Build history of the part. All positions in model axes, mm. A direction names the side the tool comes from. Round coordinates to 2 decimals unless told otherwise and drop trailing zeros. Write each loop counter-clockwise with the first axis right and the second up, starting at its lowest first coordinate (ties: lowest second). Pieces come first, ordered by that corner, then holes. Notation, with made-up numbers: (11.5, -7) - (31.5, -7) arc R35 cw to (31.5, 30) - close; hole circle Ø6 at (-32.75, 41). An arc over 180 degrees is marked (long way). Answer as a JSON object with one key per item and string values. Group by question number.
Item 1: Slice it at B-B, the plane z = -8. List the corners of the cut face in (x, y), then the cut area to 3 significant figures.
Item 2: Flat gauge pins, fed straight in: pin 1 (3 mm diameter, centred on x = 1, z = -7, fed in from +Y); pin 2 (2.5 mm diameter, centred on x = -0.5, z = -57.5, fed in from -Y); pin 3 (2 mm diameter, centred on x = 0, z = -58, fed in from -Y). Where does each tip first touch, or does it go through?
Item 3: Two-plate mould, pull along X, no slides. Class faces 4 (the cylindrical face through (0.07, 4.96, -73.7)), 5 (the flat face through (-5, 10, -41)): +X half, -X half, draft (parallel to the pull), parting line (faces both ways), or undercut.
Item 4: Slice it at A-A, the plane y = 1.25. List the corners of the cut face in (x, z), then the cut area to 3 significant figures.
Item 5: Probe line 1 (Z direction, x = 0, y = 9.25); line 2 (Y direction, x = -1.25, z = -30); line 3 (Z direction, x = 1.5, y = 9.25). List the from-to ranges inside material, lowest first. Write a range as from..to.
Item 6: Slice it at C-C, the plane x = 0. Give the number of separate pieces and of enclosed holes in the cut face, then the cut area to 3 significant figures.
Item 7: Slice it at D-D, the plane z = -30. List the corners of the cut face in (x, y).
Item 8: Which spindle directions (+Z, -Z, +X, -X, +Y, -Y) get a long thin tool onto all of the face, cutting with end or side? Do faces 1 (the cylindrical face through (0.07, 4.96, -59.7)), 2 (the cylindrical face through (0.103, 1.232, -74.348)), 3 (the flat face through (-3.44, 7.54, -37.96)). Say none if no direction does.
from build123d import *

# Parameters (mm, degrees)
SKETCH1_W           = 16
SKETCH1_H           = 80
BOSS_EXTRUDE1_DEPTH = 10
SKETCH2_R           = 2.35
CUT_EXTRUDE1_DEPTH  = 2.5
SKETCH2_3_R         = 1.7
CUT_EXTRUDE2_DEPTH  = 82.018516402
CUT_EXTRUDE3_START  = 7.5
SKETCH2_4_R         = 3
CUT_EXTRUDE3_DEPTH  = 74.518516402
SKETCH3_R           = 1.15
CUT_EXTRUDE4_DEPTH  = 83.194890352
CUT_EXTRUDE5_DEPTH  = 5
SKETCH6_R           = 2.5
CUT_EXTRUDE6_DEPTH  = 25


with BuildPart() as part:
    # Sketch1 → Boss-Extrude1 (new body)
    with BuildSketch(Plane(origin=(0, 0, 0), x_dir=(1, 0, 0), z_dir=(0, 1, 0))):
        with Locations((0, 40)):
            Rectangle(SKETCH1_W, SKETCH1_H)
    extrude(amount=BOSS_EXTRUDE1_DEPTH)

    # Sketch2 → Cut-Extrude1 (cut)
    with BuildSketch(Plane(origin=(0, 0, 0), x_dir=(1, 0, 0), z_dir=(0, 1, 0))):
        with Locations(Location((0, 72, 0), (0, 0, 270))):
            Circle(SKETCH2_R)
        with Locations(Location((0, 58, 0), (0, 0, 270))):
            Circle(SKETCH2_R)
        with Locations(Location((0, 22, 0), (0, 0, 270))):
            Circle(SKETCH2_R)
        with Locations(Location((0, 8, 0), (0, 0, 270))):
            Circle(SKETCH2_R)
    extrude(amount=CUT_EXTRUDE1_DEPTH, mode=Mode.SUBTRACT)

    # Sketch2_3 → Cut-Extrude2 (cut, through all)
    with BuildSketch(Plane(origin=(0, 0, 0), x_dir=(1, 0, 0), z_dir=(0, 1, 0))):
        with Locations(Location((0, 72, 0), (0, 0, 270))):
            Circle(SKETCH2_3_R)
        with Locations(Location((0, 58, 0), (0, 0, 270))):
            Circle(SKETCH2_3_R)
        with Locations(Location((0, 22, 0), (0, 0, 270))):
            Circle(SKETCH2_3_R)
        with Locations(Location((0, 8, 0), (0, 0, 270))):
            Circle(SKETCH2_3_R)
    extrude(amount=CUT_EXTRUDE2_DEPTH, mode=Mode.SUBTRACT)

    # Sketch2_4 → Cut-Extrude3 (cut, through all)
    with BuildSketch(Plane(origin=(0, 0, 0), x_dir=(1, 0, 0), z_dir=(0, 1, 0)).offset(CUT_EXTRUDE3_START)):
        with Locations(Location((0, 72, 0), (0, 0, 270))):
            Circle(SKETCH2_4_R)
        with Locations(Location((0, 58, 0), (0, 0, 270))):
            Circle(SKETCH2_4_R)
        with Locations(Location((0, 22, 0), (0, 0, 270))):
            Circle(SKETCH2_4_R)
        with Locations(Location((0, 8, 0), (0, 0, 270))):
            Circle(SKETCH2_4_R)
    extrude(amount=CUT_EXTRUDE3_DEPTH, mode=Mode.SUBTRACT)

    # Sketch3 → Cut-Extrude4 (cut, through all)
    with BuildSketch(Plane(origin=(8, 0, 0), x_dir=(0, 0, -1), z_dir=(1, 0, 0))):
        with Locations((30, 5)):
            Circle(SKETCH3_R)
    extrude(amount=-CUT_EXTRUDE4_DEPTH, mode=Mode.SUBTRACT)

    # Sketch4 → Cut-Extrude5 (cut)
    with BuildSketch(Plane.XZ.offset(-10)):
        Polygon((2.291567597, -44.010243295), (4.618756367, -40.020565894), (2.32718877, -36.010322599), (-2.291567597, -35.989756705), (-4.618756367, -39.979434106), (-2.32718877, -43.989677401), align=None)
    extrude(amount=CUT_EXTRUDE5_DEPTH, mode=Mode.SUBTRACT)

    # Sketch6 → Cut-Extrude6 (cut)
    with BuildSketch(Plane(origin=(0, 10, 0), x_dir=(-1, 0, 0), z_dir=(0, -1, 0))):
        with Locations(Location((0, 40, 0), (0, 0, 270))):
            Circle(SKETCH6_R)
    extrude(amount=CUT_EXTRUDE6_DEPTH, mode=Mode.SUBTRACT)


solid = part.part
Geometry says:
{
 "1": {"outline": "(-8, 0) - (-2.35, 0) - (-2.35, 2.5) - (-1.7, 2.5) - (-1.7, 7.5) - (-3, 7.5) - (-3, 10) - (-8, 10) - close; (1.7, 2.5) - (2.35, 2.5) - (2.35, 0) - (8, 0) - (8, 10) - (3, 10) - (3, 7.5) - (1.7, 7.5) - close", "area": "116 mm^2"},
 "2": {"pin 1": "stops at y = 7.5", "pin 2": "stops at y = 2.5", "pin 3": "passes through"},
 "3": {"face 4": "undercut", "face 5": "draft"},
 "4": {"outline": "(-8, -80) - (8, -80) - (8, 0) - (-8, 0) - close; hole circle Ø5 at (0, -40); hole circle Ø4.7 at (0, -72); hole circle Ø4.7 at (0, -58); hole circle Ø4.7 at (0, -22); hole circle Ø4.7 at (0, -8)", "area": "1,190 mm^2"},
 "5": {"line 1": "z = -80..-75, -69..-61, -55..-44, -36..-25, -19..-11, -5..0", "line 2": "y = 0..3.85, 6.15..10", "line 3": "z = -80..-74.6, -69.4..-60.6, -55.4..-44.01, -36.01..-24.6, -19.4..-10.6, -5.4..0"},
 "6": {"separate pieces": "6", "enclosed holes": "1", "area": "556 mm^2"},
 "7": {"outline": "(-8, 0) - (8, 0) - (8, 3.85) - (-8, 3.85) - close; (-8, 6.15) - (8, 6.15) - (8, 10) - (-8, 10) - close"},
 "8": {"face 1": "+Y, -Y", "face 2": "-Y", "face 3": "+Y"}
}
